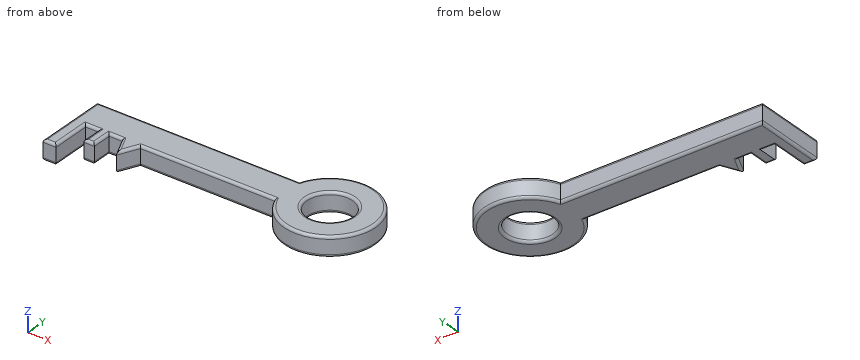
```python
from build123d import *

# Parameters (mm, degrees)
F0_R     = 17.5
F0_W     = 10
F0_H     = 30
F0_W_2   = 8
F0_H_2   = 15
F1_DEPTH = 15
F2_R     = 2
F3_R     = 2


with BuildPart() as f1:
    # F0 (on Top) → F1 (new body)
    with BuildSketch(Plane.XY):
        with BuildLine():
            Line((37.453632827, 21.7892740583), (-117.546367173, 21.7892740583))
            Line((-117.546367173, 21.7892740583), (-117.546367173, -3.2107259417))
            Line((-117.546367173, -3.2107259417), (-107.546367173, -3.2107259417))
            Line((-107.546367173, -3.2107259417), (-97.546367173, -3.2107259417))
            Line((-97.546367173, -3.2107259417), (-89.546367173, -3.2107259417))
            Line((-89.546367173, -3.2107259417), (-79.546367173, -3.2107259417))
            Line((-79.546367173, -3.2107259417), (-65.546367173, -3.2107259417))
            Line((-65.546367173, -3.2107259417), (37.453632827, -3.2107259417))
            ThreePointArc((37.453632827, -3.2107259417), (105.1453749035, 9.2892740583), (37.453632827, 21.7892740583))
        make_face()
        with Locations((70.1453749035, 9.2892740583)):
            Circle(F0_R, mode=Mode.SUBTRACT)
        with Locations((-112.546367173, -18.2107259417)):
            Rectangle(F0_W, F0_H)
        Polygon((-72.546367173, -18.2107862416), (-65.546367173, -3.2107259417), (-79.546367173, -3.2107259417), align=None)
        with Locations((-93.546367173, -10.7107259417)):
            Rectangle(F0_W_2, F0_H_2)
    extrude(amount=F1_DEPTH)

    # F2
    f2_edges = [f1.edges().sort_by_distance(p)[0] for p in [
        (-40.046367, 21.789274, 15),
        (-117.546367, -5.710726, 15),
        (-112.546367, -33.210726, 15),
        (-107.546367, -18.210726, 15),
        (-102.546367, -3.210726, 15),
        (-97.546367, -10.710726, 15),
        (-93.546367, -18.210726, 15),
        (-89.546367, -10.710726, 15),
        (-84.546367, -3.210726, 15),
        (-76.046367, -10.710756, 15),
        (-69.046367, -10.710756, 15),
        (-14.046367, -3.210726, 15),
        (105.145375, 9.289274, 15),
        (52.645375, 9.289274, 15),
    ]]
    fillet(f2_edges, radius=F2_R)

    # F3
    f3_edges = [f1.edges().sort_by_distance(p)[0] for p in [
        (105.145375, 9.289274, 0),
        (52.645375, 9.289274, 0),
        (-40.046367, 21.789274, 0),
        (-14.046367, -3.210726, 0),
        (-69.046367, -10.710756, 0),
        (-89.546367, -10.710726, 0),
        (-93.546367, -18.210726, 0),
        (-107.546367, -18.210726, 0),
        (-117.546367, -5.710726, 0),
        (-112.546367, -33.210726, 0),
        (-102.546367, -3.210726, 0),
        (-76.046367, -10.710756, 0),
        (-84.546367, -3.210726, 0),
    ]]
    fillet(f3_edges, radius=F3_R)


solid = f1.part
```
Check sheet for the modelled part. Datum: model origin and axes. Units: mm. Give positions to 0.01 mm unless a question says otherwise; leave off trailing zeros. Write each loop counter-clockwise with the first axis right and the second up, starting at its lowest first coordinate (ties: lowest second). Pieces come first, ordered by that corner, then holes.
Item 1: Cross-section at A-A (x = -51). Enter the section's corners in (y, z).
Item 2: Gauge pin test, flat ends, axial feed: pin 1 (10 mm diameter, centred on x = -74.5, y = -18.5, fed in from -Z); pin 2 (3.5 mm diameter, centred on y = -8.5, z = 7.5, fed in from +X); pin 3 (6.5 mm diameter, centred on x = -94.5, z = 5, fed in from -Y); pin 4 (12 mm diameter, centred on x = 66.5, y = -0.5, fed in from +Z). Record the tip position at first contact, or that the pin passes through.
Item 3: Scan lines: L1, parallel to X at y = -17, z = 14.25; L2, parallel to X at y = -3.5, z = 13.25; L3, parallel to Y at x = -17, z = 10.5. Record each from-to range of solid material in increasing order.
Item 4: Cross-section at B-B (z = 8.25). Enter the section's corners in (x, y).
Report:
1. outline: (-3.21, 2) arc R2 ccw to (-1.21, 0) - (19.79, 0) arc R2 ccw to (21.79, 2) - (21.79, 13) arc R2 ccw to (19.79, 15) - (-1.21, 15) arc R2 ccw to (-3.21, 13) - close
2. pin 1: stops at z = 0.01
2. pin 2: stops at x = 101.25
2. pin 3: stops at y = -18.21
2. pin 4: passes through
3. L1: x = -117.11 to -107.99, -97.11 to -89.99, -72.63 to -72.47, 47.71 to 92.58
3. L2: x = -117.53 to -107.56, -97.53 to -89.56, -79.39 to -65.7, 37.58 to 58.18, 82.11 to 102.71
3. L3: y = -3.21 to 21.79
4. outline: (-117.55, -33.21) - (-107.55, -33.21) - (-107.55, -3.21) - (-97.55, -3.21) - (-97.55, -18.21) - (-89.55, -18.21) - (-89.55, -3.21) - (-79.55, -3.21) - (-72.55, -18.21) - (-65.55, -3.21) - (37.45, -3.21) arc R35 ccw (long way) to (37.45, 21.79) - (-117.55, 21.79) - close; hole circle Ø35 at (70.15, 9.29)
